Check sheet for the drawn part. Datum: minimum x, y, z corner. Units: mm. A direction names the side the tool comes from. Coordinates: 2 decimals unless noted, no trailing zeros. Write each loop counter-clockwise with the first axis right and the second up, starting at its lowest first coordinate (ties: lowest second). Pieces come first, ordered by that corner, then holes. Notation, with made-up numbers: M -24,-1 L 7,-1 A23 cw 7,15 Z; hole C 86,75.5 d6. An arc over 180 degrees is marked long. Answer as a JSON object with one key per item and string values. Group by question number.
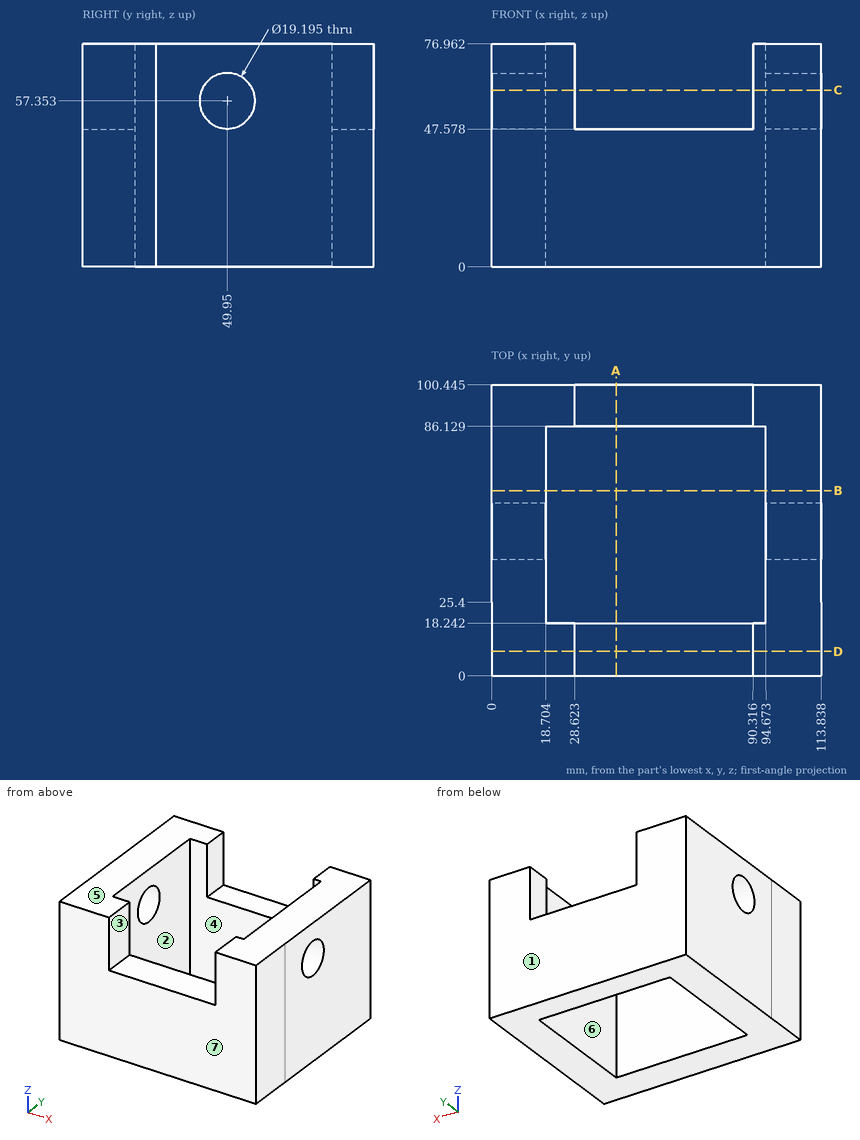
1) Draft check along Y on the marked faces 4, 5, 6 and 7. Enter one of: +Y half, -Y half, draft (parallel to the pull), parting line (faces both ways), or undercut.
2) Section check D-D (y = 8.5). Record the cut outline in (x, z), then the cut area to 3 significant figures.
3) Section check B-B (y = 64). Record the cut outline in (x, z), then the cut area to 3 significant figures.
4) Material ranges on probe 1 along X at (y, z) = (31, 55); probe 2 along Y at (x, z) = (72, 27) (1 decimal); probe 3 along Z at (x, y) = (80, 17.5), recorded low to high. Write a range as [from, to].
5) Section check A-A (x = 43). Record the cut outline in (y, z) (1 decimal).
6) Section check C-C (z = 61). State how many separate pieces and enclosed holes the cut face has, then the cut area to 3 significant figures.
7) Go/stop test with flat-tipped pins: pin 1 Ø11.5 at (y, z) = (49.95, 57.35) entering from +X; pin 2 Ø12 at (x, z) = (66, 39.5) entering from -Y; pin 3 Ø4.5 at (x, y) = (60.5, 93.5) entering from +Z. Record where each tip stops, or that it passes through.
8) Set-up check for the marked faces 1, 2 and 3: record each of +Z, -Z, +X, -X, +Y, -Y from which the full face is reachable in a straight line by a thin tool's end or side.
Entries:
{
 "1": {"face 4": "undercut", "face 5": "draft", "face 6": "undercut", "face 7": "-Y half"},
 "2": {"outline": "M 0,0 L 113.84,0 L 113.84,76.96 L 90.32,76.96 L 90.32,47.58 L 28.62,47.58 L 28.62,76.96 L 0,76.96 Z", "area": "6,950 mm^2"},
 "3": {"outline": "M 0,0 L 18.7,0 L 18.7,76.96 L 0,76.96 Z; M 94.67,0 L 113.84,0 L 113.84,76.96 L 94.67,76.96 Z", "area": "2,910 mm^2"},
 "4": {"probe 1": "[0, 18.7], [94.67, 113.84]", "probe 2": "[0, 18.2], [86.1, 100.4]", "probe 3": "[0, 47.58]"},
 "5": {"outline": "M 0,0 L 18.2,0 L 18.2,47.6 L 0,47.6 Z; M 86.1,0 L 100.4,0 L 100.4,47.6 L 86.1,47.6 Z"},
 "6": {"separate pieces": "4", "enclosed holes": "0", "area": "3,600 mm^2"},
 "7": {"pin 1": "through", "pin 2": "y = 0", "pin 3": "z = 47.58"},
 "8": {"face 1": "+Z, -Z, +X, -X, +Y", "face 2": "+Z, -Z", "face 3": "+Z, +Y, -Y"}
}
